Verification items for the finished model (mm, model axes). Round coordinates to 2 decimals unless told otherwise and drop trailing zeros. Order: outer loops, then holes, each group sorted by start corner. A loop starts at its lowest first (then second) coordinate and runs counter-clockwise, first axis right, second up. Notation, with made-up numbers: (37.25, 56.5) -> (73.25, 56.5) arc R20 cw to (73.25, 68.5) -> close; hole circle Ø10 at (87, 27.25). An arc over 180 degrees is marked (long way). Return JSON: item names as keys, results as strings. Group by question number.
1) Section check C-C on z = 2.7. State how many separate pieces and enclosed holes the cut face has, plus the area to 3 significant figures.
2) Scan lines: L1, parallel to Y at x = 1025, z = 0.65; L2, parallel to X at y = 147, z = 1; L3, parallel to Y at x = 1024, z = 3.4. Record each from-to range of solid material in increasing order.
3) Section check A-A on y = 43. Enter the section's corners in (x, z) (3 decimals).
4) Depth check by flat-ended pin: pin 1 (3 mm diameter, centred on x = 973.5, z = 2.5, fed in from -Y); pin 2 (1 mm diameter, centred on x = 965.5, z = 1.5, fed in from +Y). Enter the tip coordinate at first touch or a pass-through.
5) Section check B-B on y = 207.5. Enter the section's corners in (x, z) (3 decimals), plus the area to 3 significant figures.
```python
from build123d import *

# Parameters (mm, degrees)
BOSS_EXTRUDE1_DEPTH   = 5.715
F_6_CLEARANCE_HOLE1_D = 3.7973


with BuildPart() as part:
    # Model → Boss-Extrude1 (new body)
    with BuildSketch(Plane.XY):
        Polygon((953.262, 22.8575), (964.099, 22.8575), (964.099, 28.5722), (975.526, 28.5722), (975.526, 22.8575), (986.956, 22.8575), (986.956, 28.5722), (998.386, 28.5722), (998.386, 22.8575), (1009.82, 22.8575), (1009.82, 28.5722), (1021.25, 28.5722), (1021.25, 22.8575), (1032.08, 22.8575), (1032.08, 28.5722), (1032.08, 288.572), (1032.08, 294.287), (1021.25, 294.287), (1021.25, 288.572), (1009.82, 288.572), (1009.82, 294.287), (998.386, 294.287), (998.386, 288.572), (986.956, 288.572), (986.956, 294.287), (975.526, 294.287), (975.526, 288.572), (964.099, 288.572), (964.099, 294.287), (953.262, 294.287), (953.262, 288.572), (953.262, 265.712), (953.262, 265.339), (953.361, 264.218), (953.654, 262.755), (954.133, 261.342), (954.606, 260.321), (954.793, 259.997), (954.888, 259.836), (955.192, 259.36), (955.626, 258.753), (956.098, 258.175), (956.61, 257.631), (957.153, 257.121), (957.732, 256.647), (958.338, 256.211), (958.815, 255.907), (958.977, 255.814), (959.139, 255.721), (959.612, 255.418), (960.222, 254.981), (960.801, 254.507), (961.344, 253.997), (961.856, 253.453), (962.328, 252.876), (962.766, 252.268), (963.069, 251.792), (963.161, 251.63), (963.348, 251.307), (963.824, 250.286), (964.304, 248.874), (964.593, 247.41), (964.692, 246.29), (964.692, 245.915), (964.692, 71.2294), (964.692, 70.8561), (964.593, 69.7357), (964.304, 68.272), (963.824, 66.8595), (963.348, 65.8386), (963.161, 65.5147), (963.069, 65.3535), (962.766, 64.878), (962.328, 64.2705), (961.856, 63.693), (961.344, 63.1486), (960.801, 62.6389), (960.222, 62.1647), (959.612, 61.728), (959.139, 61.4246), (958.977, 61.3311), (958.815, 61.2373), (958.338, 60.9353), (957.732, 60.4986), (957.153, 60.0244), (956.61, 59.5147), (956.098, 58.9703), (955.626, 58.3928), (955.192, 57.7854), (954.888, 57.3098), (954.793, 57.1472), (954.606, 56.8247), (954.133, 55.8038), (953.654, 54.3913), (953.361, 52.9276), (953.262, 51.8072), (953.262, 51.4325), (953.262, 28.5722), align=None)
        Polygon((970.407, 272.872), (970.407, 278.587), (976.122, 278.587), (976.122, 267.158), (970.407, 267.158), align=None, mode=Mode.SUBTRACT)
        Polygon((970.407, 250.012), (970.407, 255.728), (976.122, 255.728), (976.122, 244.297), (970.407, 244.297), align=None, mode=Mode.SUBTRACT)
        Polygon((970.407, 227.153), (970.407, 232.868), (976.122, 232.868), (976.122, 221.437), (970.407, 221.437), align=None, mode=Mode.SUBTRACT)
        Polygon((970.407, 204.293), (970.407, 210.008), (976.122, 210.008), (976.122, 198.578), (970.407, 198.578), align=None, mode=Mode.SUBTRACT)
        Polygon((970.407, 181.433), (970.407, 187.147), (976.122, 187.147), (976.122, 175.718), (970.407, 175.718), align=None, mode=Mode.SUBTRACT)
        Polygon((970.407, 158.572), (970.407, 164.287), (976.122, 164.287), (976.122, 152.858), (970.407, 152.858), align=None, mode=Mode.SUBTRACT)
        Polygon((970.407, 135.712), (970.407, 141.428), (976.122, 141.428), (976.122, 129.997), (970.407, 129.997), align=None, mode=Mode.SUBTRACT)
        Polygon((970.407, 112.853), (970.407, 118.568), (976.122, 118.568), (976.122, 107.137), (970.407, 107.137), align=None, mode=Mode.SUBTRACT)
        Polygon((970.407, 89.9929), (970.407, 95.7076), (976.122, 95.7076), (976.122, 84.2779), (970.407, 84.2779), align=None, mode=Mode.SUBTRACT)
        Polygon((970.407, 67.1326), (970.407, 72.8472), (976.122, 72.8472), (976.122, 61.4179), (970.407, 61.4179), align=None, mode=Mode.SUBTRACT)
        Polygon((970.407, 44.2722), (970.407, 49.9868), (976.122, 49.9868), (976.122, 38.5576), (970.407, 38.5576), align=None, mode=Mode.SUBTRACT)
    extrude(amount=BOSS_EXTRUDE1_DEPTH)

    # #6 Clearance Hole1 (through all)
    with Locations(Plane.XY.offset(5.715)):
        with Locations((1025.122, 284.072), (995.122, 284.072), (980.622, 269.572), (980.622, 219.713875), (980.622, 169.85575), (980.622, 147.28845), (980.622, 97.430325), (980.622, 47.5722), (995.122, 33.0722), (1025.122, 33.0722)):
            Hole(F_6_CLEARANCE_HOLE1_D / 2)


solid = part.part
```
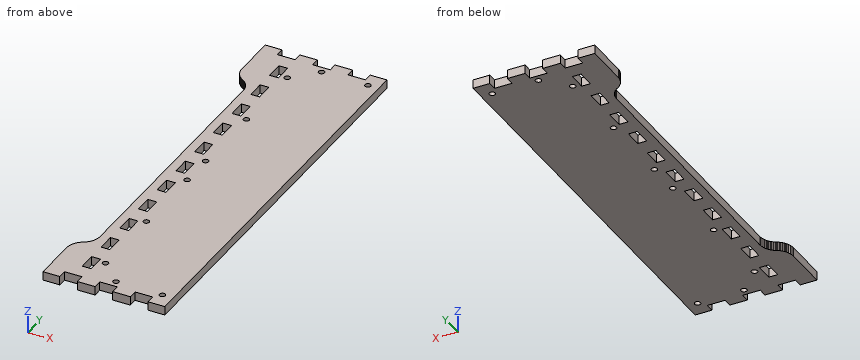
Check result:
{
 "1": {"separate pieces": "1", "enclosed holes": "21", "area": "17,900 mm^2"},
 "2": {"L1": "22.86 to 31.18, 34.97 to 282.18, 285.97 to 294.29", "L2": "964.69 to 978.75, 982.5 to 1032.08", "L3": "22.86 to 31.54, 34.6 to 282.54, 285.6 to 294.29"},
 "3": {"outline": "(953.262, 0) -> (970.407, 0) -> (970.407, 5.715) -> (953.262, 5.715) -> close; (976.122, 0) -> (1032.08, 0) -> (1032.08, 5.715) -> (976.122, 5.715) -> close"},
 "4": {"pin 1": "y = 28.57", "pin 2": "y = 288.57"},
 "5": {"outline": "(964.692, 0) -> (970.407, 0) -> (970.407, 5.715) -> (964.692, 5.715) -> close; (976.122, 0) -> (1032.08, 0) -> (1032.08, 5.715) -> (976.122, 5.715) -> close", "area": "352 mm^2"}
}
